from build123d import *

# Parameters (mm, degrees)
RESSALTO_EXTRUS_O1_DEPTH = 57
CORTE_EXTRUS_O1_DEPTH    = 18.5


with BuildPart() as part:
    # Esboço1 → Ressalto-extrusão1 (new body)
    with BuildSketch(Plane(origin=(0, 0, 0), x_dir=(1, 0, 0), z_dir=(0, 1, 0))):
        with BuildLine():
            Line((-72, 0), (72, 0))
            ThreePointArc((72, 0), (72.85009345, 3.078711179), (75.159487509, 5.285024956))
            ThreePointArc((75.159487509, 5.285024956), (77.004661638, 4.729916917), (76.449553599, 2.884742789))
            ThreePointArc((76.449553599, 2.884742789), (77.536782743, -3.242075689), (80.296246294, 2.335139815))
            ThreePointArc((80.296246294, 2.335139815), (81.096189798, 3.978813584), (82.863892701, 3.513196237))
            ThreePointArc((82.863892701, 3.513196237), (83.342245662, -2.731375348), (78, -6))
            Line((78, -6), (-78, -6))
            ThreePointArc((-78, -6), (-83.342245662, -2.731375348), (-82.863892701, 3.513196237))
            ThreePointArc((-82.863892701, 3.513196237), (-81.096189798, 3.978813584), (-80.296246294, 2.335139815))
            ThreePointArc((-80.296246294, 2.335139815), (-77.536782743, -3.242075689), (-76.449553599, 2.884742789))
            ThreePointArc((-76.449553599, 2.884742789), (-77.004661638, 4.729916917), (-75.159487509, 5.285024956))
            ThreePointArc((-75.159487509, 5.285024956), (-72.85009345, 3.078711179), (-72, 0))
        make_face()
    extrude(amount=RESSALTO_EXTRUS_O1_DEPTH)

    # Esboço3 → Corte-extrusão1 (cut, symmetric)
    with BuildSketch(Plane(origin=(0, 28.5, 0), x_dir=(1, 0, 0), z_dir=(0, 1, 0))):
        with BuildLine():
            Line((-72, 0), (-72, -6))
            Line((-72, -6), (-78, -6))
            ThreePointArc((-78, -6), (-82.242640687, 4.242640687), (-72, 0))
        make_face()
        with BuildLine():
            Line((72, 0), (72, -6))
            Line((72, -6), (78, -6))
            ThreePointArc((78, -6), (82.242640687, 4.242640687), (72, 0))
        make_face()
    extrude(amount=CORTE_EXTRUS_O1_DEPTH, both=True, mode=Mode.SUBTRACT)


solid = part.part
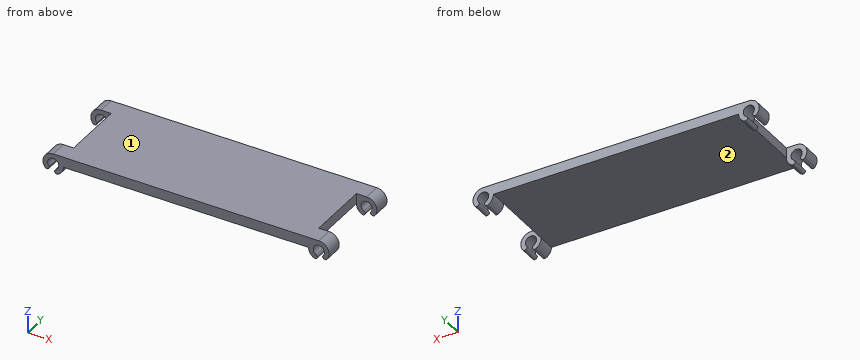
Part model, mm, in its own coordinate system. Face numbers are marked on the shaded views. Coordinates: 2 decimals unless noted, no trailing zeros. Write each loop counter-clockwise with the first axis right and the second up, starting at its lowest first coordinate (ties: lowest second). Pieces come first, ordered by that corner, then holes. Notation, with made-up numbers: (-10.5, -7) - (35.5, -7) arc R33 ccw to (35.5, 22) - close; hole circle Ø4 at (79, -25). An arc over 180 degrees is marked (long way). Put each result on its own line as item: value.
1. Two-plate mould, pull along X, no slides. Class the marked faces 1 and 2: +X half, -X half, draft (parallel to the pull), parting line (faces both ways), or undercut.
Final values:
face 1: draft
face 2: undercut
2. Band-saw the part on A-A (x = -39). Write the cut outline in (y, z).
Final values:
outline: (0, 0) - (57, 0) - (57, 6) - (0, 6) - close
3. Flat gauge pins, fed straight in: pin 1 Ø12 at (x, y) = (-4.5, 30.5) entering from -Z; pin 2 Ø6.5 at (y, z) = (35.5, 4) entering from +X; pin 3 Ø1.8 at (y, z) = (25, 2.5) entering from -X. Where does each tip first touch, or does it go through?
Final values:
pin 1: stops at z = 0
pin 2: stops at x = 72
pin 3: stops at x = -72
4. Probe line 1 along Z through (x, y) = (-13, 26); line 2 along Z through (x, y) = (78, 50.25) (3 decimals); line 3 along Y through (x, z) = (-72.5, -1). List the from-to ranges inside material, lowest first. Write a range as [from, to].
Final values:
line 1: z = [0, 6]
line 2: z = [3.275, 6]
line 3: y = [0, 10], [47, 57]
